```python
from build123d import *

# Parameters (mm, degrees)
SKETCH_W        = 77
SKETCH_H        = 26
PAD_DEPTH       = 19
SKETCH001_R     = 2.875
POCKET_DEPTH    = 17
POCKET001_DEPTH = 8


with BuildPart() as part:
    # Sketch → Pad (new body)
    with BuildSketch(Plane.XY):
        with Locations((17.5, 0)):
            Rectangle(SKETCH_W, SKETCH_H)
    extrude(amount=PAD_DEPTH)

    # Sketch001 (on Face6 of Pad) → Pocket (cut)
    with BuildSketch(Plane.XY.offset(19)):
        with Locations((-9.75, 0)):
            Circle(SKETCH001_R)
        with Locations((9.75, 0)):
            Circle(SKETCH001_R)
    extrude(amount=-POCKET_DEPTH, mode=Mode.SUBTRACT)

    # Sketch002 (on Face5 of Pocket) → Pocket001 (cut)
    with BuildSketch(Plane.XY.offset(19)):
        with BuildLine():
            Line((44, 3), (50, 3))
            ThreePointArc((50, -3), (53, 0), (50, 3))
            Line((44, -3), (50, -3))
            ThreePointArc((44, 3), (41, 0), (44, -3))
        make_face()
    extrude(amount=-POCKET001_DEPTH, mode=Mode.SUBTRACT)


solid = part.part
```
Geometry check sheet. Reference: the model listing, model coordinates, mm. A direction names the side the tool comes from. Round coordinates to 2 decimals unless told otherwise and drop trailing zeros. Order: outer loops, then holes, each group sorted by start corner. A loop starts at its lowest first (then second) coordinate and runs counter-clockwise, first axis right, second up. Notation, with made-up numbers: (5.5, -14) - (52.5, -14) arc R17 cw to (52.5, 8) - close; hole circle Ø3 at (67, -26.75). An arc over 180 degrees is marked (long way). Use a Markdown table: item, result. Add a question column.
(1) Material ranges on line 1 along Y through (x, z) = (-9.75, 12) (3 decimals); line 2 along X through (y, z) = (-1.25, 9); line 3 along Y through (x, z) = (52, 17.25), recorded low to high. Write a range as [from, to].
(2) Sectioned sample at A-A, the plane x = -9.75. Enter the section's corners in (y, z) (3 decimals), and give its area (3 significant figures).
(3) Sectioned sample at B-B, the plane y = 0. Enter the section's corners in (x, z) (3 decimals).
(4) Release check for a two-part mould opening along X. For faces 3 (the flat face through (56, 0, 9)), 4 (the flat face through (17, 0, 19)), 5 (the cylindrical face through (53, 0, 15)) record: pulls with the +X half, pulls with the -X half, needs draft (parallel to the pull), parting line crosses it, or undercut.
(5) Tool access check on faces 1 (the cylindrical face through (-12.622, 0.126, 10.619)), 2 (the flat face through (-21, 0, 9)). Record the directions out of +Z, -Z, +X, -X, +Y, -Y that give a thin tool (end or side, any length) a straight path to the whole face; none if there is none.
(6) Sectioned sample at C-C, the plane x = 48. Enter the section's corners in (y, z), and give its area (3 significant figures).
(7) Depth check by flat-ended pin: pin 1 (3.5 mm diameter, centred on x = 9.75, y = 0, fed in from +Z); pin 2 (3 mm diameter, centred on x = 45.5, y = -0.5, fed in from +Z). Enter the tip coordinate at first touch or a pass-through.
Answers below:
| question | item | result |
|---|---|---|
| 1 | line 1 | [-13, -2.875], [2.875, 13] |
| 1 | line 2 | [-21, -12.34], [-7.16, 7.16], [12.34, 56] |
| 1 | line 3 | [-13, -2.24], [2.24, 13] |
| 2 | outline | (-13, 0) - (13, 0) - (13, 19) - (2.875, 19) - (2.875, 2) - (-2.875, 2) - (-2.875, 19) - (-13, 19) - close |
| 2 | area | 396 mm² |
| 3 | outline | (-21, 0) - (56, 0) - (56, 19) - (53, 19) - (53, 11) - (41, 11) - (41, 19) - (12.625, 19) - (12.625, 2) - (6.875, 2) - (6.875, 19) - (-6.875, 19) - (-6.875, 2) - (-12.625, 2) - (-12.625, 19) - (-21, 19) - close |
| 4 | face 3 | pulls with the +X half |
| 4 | face 4 | needs draft |
| 4 | face 5 | undercut |
| 5 | face 1 | +Z |
| 5 | face 2 | +Z, -Z, -X, +Y, -Y |
| 6 | outline | (-13, 0) - (13, 0) - (13, 19) - (3, 19) - (3, 11) - (-3, 11) - (-3, 19) - (-13, 19) - close |
| 6 | area | 446 mm² |
| 7 | pin 1 | z = 2 |
| 7 | pin 2 | z = 11 |
